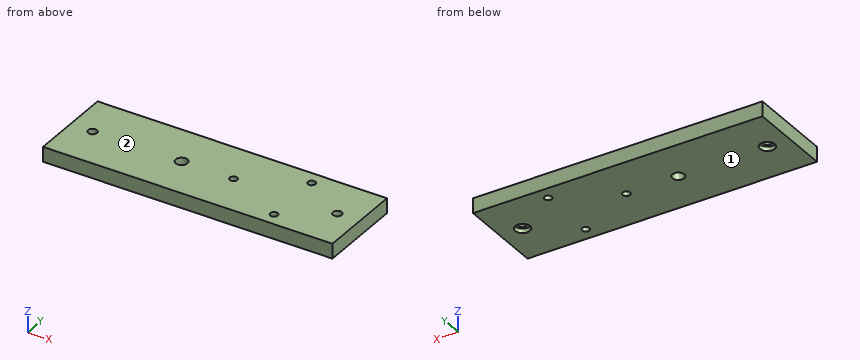
Autodesk Inventor part; units mm, degrees
ref_plane "YZ Plane" through (0, 0, 0) normal (1, 0, 0) x (0, 1, 0)
ref_plane "XZ Plane" through (0, 0, 0) normal (0, 1, 0) x (-1, 0, 0)
ref_plane "XY Plane" through (0, 0, 0) normal (0, 0, 1) x (1, 0, 0)
sketch "Sketch1" plane through (0, 0, 0) normal (0, 0, 1) x (1, 0, 0)
  line L0 (-57.5, 29) -> (57.5, 29)
  line L1 (57.5, 29) -> (57.5, -29)
  line L2 (57.5, -29) -> (-57.5, -29)
  line L3 (-57.5, -29) -> (-57.5, 29)
  circle A0 centre (12.5, 0) radius 2.5
  circle A1 centre (52.5, 20) radius 2.5
  circle A2 centre (52.5, -20) radius 2.5
  circle A3 centre (-22.5, 0) radius 4
  point P0 (0, 0)
  dimension "d0" = 115
  dimension "d1" = 58
  dimension "d2" = 29
  dimension "d3" = 57.5
  dimension "d4" = 5
  dimension "d5" = 45
  dimension "d6" = 29
  dimension "d7" = 5
  dimension "d8" = 5
  dimension "d9" = 5
  dimension "d11" = 5
  dimension "d13" = 8
  dimension "d14" = 80
  dimension "d15" = 29
  dimension "d18" = 40
  dimension "d19" = 20
  dimension "d20" = 20
extrude "Extrusion1" add sketch "Sketch1" along normal blind 10
sketch "Sketch3" plane through (-57.5, -29, 0) normal (-1, 0, 0) x (0, 0, 1)
  line L0 (0, 0) -> (0, 58)
  line L1 (0, 0) -> (10, 0)
  line L2 (10, 58) -> (10, 0)
  line L3 (0, 58) -> (10, 58)
  point P0 (0, 29)
extrude "Extrusion2" add sketch "Sketch3" along normal blind 40
sketch "Sketch4" plane through (57.5, -29, 0) normal (1, 0, 0) x (0, 0, -1)
  line L0 (0, 58) -> (0, 0)
  line L1 (0, 58) -> (-10, 58)
  line L2 (-10, 0) -> (-10, 58)
  line L3 (0, 0) -> (-10, 0)
  point P0 (0, 29)
extrude "Extrusion3" add sketch "Sketch4" along normal blind 40
hole "Hole1" at (82.5, 0, 0) direction (0, 0, 1) diameter 6 end through all counterbore diameter 10 counterbore depth 3
hole "Hole2" at (-82.5, 0, 0) direction (0, 0, 1) diameter 6 end through all counterbore diameter 10 counterbore depth 3
equation "\"d6\" = 0.5 * d1"
equation "\"d11\" = d9"
equation "\"d15\" = 0.5 * d1"
properties part number "suport maneta vid"
For this review, take the finished solid that the model builds, in its own axes (mm). Face numbers are marked on the shaded views. Round coordinates to 2 decimals unless told otherwise and drop trailing zeros. Loops run counter-clockwise (first coordinate to the right, second up) from the corner with the lowest first, then second, coordinate; pieces in that order, holes last. Notation, with made-up numbers: (1, 41) - (47, 41) arc R27 cw to (47, 65) - close; hole circle Ø8 at (58, 12). An arc over 180 degrees is marked (long way). Use one line per item in the form item = value.
Item 1: Clearance check with flat-ended pins moving along their axes: P1, Ø5, axis at x = -22.5, y = 0, coming from the -Z side; P2, Ø9.5, axis at x = -82.5, y = 0, coming from the -Z side. State where each tip first meets the part, or that it passes through.
Answers:
P1 = through
P2 = 3
Item 2: Consider section B-B on x = 52.5. Write out the cut boundary in (y, z).
Answers:
outline = (-29, 0) - (-22.5, 0) - (-22.5, 10) - (-29, 10) - close; (-17.5, 0) - (17.5, 0) - (17.5, 10) - (-17.5, 10) - close; (22.5, 0) - (29, 0) - (29, 10) - (22.5, 10) - close
Item 3: Consider section D-D on x = -22.5. Write out the cut boundary in (y, z), then the cut area to 3 significant figures.
Answers:
outline = (-29, 0) - (-4, 0) - (-4, 10) - (-29, 10) - close; (4, 0) - (29, 0) - (29, 10) - (4, 10) - close
area = 500 mm^2
Item 4: Mouldability with a two-part tool opening along Z and no side actions: class the marked faces 1 and 2 as +Z half, -Z half, draft (parallel to the pull), parting line (faces both ways), or undercut.
Answers:
face_1 = -Z half
face_2 = +Z half
Item 5: For line 1 (Y direction, x = 52.5, z = 2.75); line 2 (Y direction, x = -82.5, z = 1.45); line 3 (X direction, y = -0.5, z = 5.25), list the stretches that pass through material, from the lowest coordinate up.
Answers:
line_1 = -29 to -22.5, -17.5 to 17.5, 22.5 to 29
line_2 = -29 to -5, 5 to 29
line_3 = -97.5 to -85.46, -79.54 to -26.47, -18.53 to 10.05, 14.95 to 79.54, 85.46 to 97.5
Item 6: Consider section C-C on y = 0. Write out the cut boundary in (x, z), then the cut area to 3 significant figures.
Answers:
outline = (-97.5, 0) - (-87.5, 0) - (-87.5, 3) - (-85.5, 3) - (-85.5, 10) - (-97.5, 10) - close; (-79.5, 3) - (-77.5, 3) - (-77.5, 0) - (-26.5, 0) - (-26.5, 10) - (-79.5, 10) - close; (-18.5, 0) - (10, 0) - (10, 10) - (-18.5, 10) - close; (15, 0) - (77.5, 0) - (77.5, 3) - (79.5, 3) - (79.5, 10) - (15, 10) - close; (85.5, 3) - (87.5, 3) - (87.5, 0) - (97.5, 0) - (97.5, 10) - (85.5, 10) - close
area = 1,680 mm^2
Item 7: Consider section A-A on y = -20. Write out the cut boundary in (x, z), then the cut area to 3 significant figures.
Answers:
outline = (-97.5, 0) - (50, 0) - (50, 10) - (-97.5, 10) - close; (55, 0) - (97.5, 0) - (97.5, 10) - (55, 10) - close
area = 1,900 mm^2
